Work out the finished part from the listing and answer in its coordinate system (mm). A direction names the side the tool comes from. Coordinates: 2 decimals unless noted, no trailing zeros. Loops run counter-clockwise (first coordinate to the right, second up) from the corner with the lowest first, then second, coordinate; pieces in that order, holes last. Notation, with made-up numbers: (61, 50) - (94, 50) arc R11 cw to (94, 70) - close; hole circle Ø8 at (88, -35.5). An arc over 180 degrees is marked (long way). Write each question's results on one line, items separated by ' | '. Start each with the question number.
Item 1: Section D-D, the plane y = 33.5 is taken. Write down the section's boundary in (x, z), plus the area to 3 significant figures.
Item 2: Section C-C, the plane x = -9 is taken. Write down the section's boundary in (y, z).
Item 3: Each of these flat-tipped pins is pushed along its axis until it touches: pin 1 Ø1.5 at (x, y) = (-3.5, -5.5) entering from -Z; pin 2 Ø4 at (x, y) = (0, 0) entering from +Z; pin 3 Ø1 at (x, z) = (-14.5, 3) entering from +Y; pin 4 Ø1.5 at (y, z) = (21.5, 3) entering from -X. Where does it stop, or does it pass through?
Item 4: For a pull along Y with two mould halves and no side action, classify faces 1 (the face through (0, 50, 0)), 2 (the face through (-14, -28.12, 3)), 3 (the face through (-2.476, -18.539, 1.894)) as +Y half, -Y half, draft (parallel to the pull), parting line (faces both ways), or undercut.
Item 5: Consider probe 1 along Y at (x, z) = (0, 3.2); probe 2 along Z at (x, y) = (-3, 1); probe 3 along Y at (x, z) = (-18.5, 2.05). Determine where each line is inside the solid, lowest interval first. Write a range as [from, to].
Item 6: Section A-A, the plane y = 0 is taken. Write down the section's boundary in (x, z), plus the area to 3 significant figures.
Item 7: Section B-B, the plane z = 3.4 is taken. Write down the section's boundary in (x, y).
Item 8: A tool of negligible diameter and unlimited length cuts with its end or side. For faces 4 (the face through (4, -17, 2.3)), 5 (the face through (-0.1, 9.1, 1.2)), 6 (the face through (-6.5, 31, 2)), from which of +Z, -Z, +X, -X, +Y, -Y can it reach the whole face along a straight path? Write none if from no direction.
from build123d import *

# Parameters (mm, degrees)
SKETCH1_W           = 27
SKETCH1_H           = 4
SKETCH1_W_2         = 13
SKETCH1_R           = 6.5
SKETCH1_R_2         = 2.5
BOSS_EXTRUDE1_DEPTH = 5
SKETCH2_R           = 2.5
CUT_EXTRUDE1_DEPTH  = 1.5
CUT_EXTRUDE2_DEPTH  = 0.8
FILLET1_R           = 1


with BuildPart() as part:
    # Sketch1 → Boss-Extrude1 (new body)
    # profile 1 of 6: a face of its own
    with BuildSketch(Plane.XY):
        with Locations((-20, -26.12)):
            Rectangle(SKETCH1_W, SKETCH1_H)
    # profile 2 of 6: a face of its own
    with BuildSketch(Plane.XY):
        with Locations((0, -26.12)):
            Rectangle(SKETCH1_W_2, SKETCH1_H)
    # profile 3 of 6: a face of its own
    with BuildSketch(Plane.XY):
        with BuildLine():
            Line((-6.5, -24.12), (6.5, -24.12))
            Line((6.5, -24.12), (6.5, 0))
            ThreePointArc((6.5, 0), (0, -6.5), (-6.5, 0))
            Line((-6.5, 0), (-6.5, -24.12))
        make_face()
    # profile 4 of 6: a face of its own
    with BuildSketch(Plane.XY):
        Circle(SKETCH1_R)
        Circle(SKETCH1_R_2, mode=Mode.SUBTRACT)
    # profile 5 of 6: a face of its own
    with BuildSketch(Plane.XY):
        with BuildLine():
            ThreePointArc((-6.5, 0), (0, 6.5), (6.5, 0))
            Line((6.5, 0), (6.5, 84.43))
            ThreePointArc((6.5, 84.43), (0, 77.93), (-6.5, 84.43))
            Line((-6.5, 84.43), (-6.5, 0))
        make_face()
    # profile 6 of 6: a face of its own
    with BuildSketch(Plane.XY):
        with Locations((0, 84.43)):
            Circle(SKETCH1_R)
        with Locations((0, 84.43)):
            Circle(SKETCH1_R_2, mode=Mode.SUBTRACT)
    extrude(amount=BOSS_EXTRUDE1_DEPTH)

    # Sketch2 → Cut-Extrude1 (cut)
    with BuildSketch(Plane(origin=(0, 0, 0), x_dir=(-1, 0, 0), z_dir=(0, 0, -1))):
        with BuildLine():
            Line((33.5, -28.12), (33.5, -24.12))
            Line((33.5, -24.12), (6.5, -24.12))
            Line((6.5, -24.12), (6.5, 6.368673331))
            ThreePointArc((6.5, 6.368673331), (0, 9.1), (-6.5, 6.368673331))
            Line((-6.5, 6.368673331), (-6.5, -28.12))
            Line((-6.5, -28.12), (33.5, -28.12))
        make_face()
        Circle(SKETCH2_R, mode=Mode.SUBTRACT)
    extrude(amount=-CUT_EXTRUDE1_DEPTH, mode=Mode.SUBTRACT)

    # Sketch3 → Cut-Extrude2 (cut)
    with BuildSketch(Plane(origin=(0, 0, 1.5), x_dir=(-1, 0, 0), z_dir=(0, 0, -1))):
        with BuildLine():
            ThreePointArc((-0.425, -16.56), (-1.318324317, -14.403324317), (-3.475, -13.51))
            ThreePointArc((-3.475, -13.51), (-5.489184715, -14.269681259), (-6.5, -16.170288568))
            Line((-6.5, -16.170288568), (-6.5, -16.949711432))
            ThreePointArc((-6.5, -16.949711432), (-5.489184715, -18.850318741), (-3.475, -19.61))
            ThreePointArc((-3.475, -19.61), (-1.318324317, -18.716675683), (-0.425, -16.56))
        make_face()
        with BuildLine():
            Line((-6.5, -16.949711432), (-6.5, -16.170288568))
            ThreePointArc((-6.5, -16.170288568), (-6.525, -16.56), (-6.5, -16.949711432))
        make_face()
        with BuildLine():
            Line((-6.5, -19.61), (-3.475, -19.61))
            ThreePointArc((-3.475, -19.61), (-5.489184715, -18.850318741), (-6.5, -16.949711432))
            Line((-6.5, -16.949711432), (-6.5, -19.61))
        make_face()
        with BuildLine():
            ThreePointArc((-6.5, -16.170288568), (-5.489184715, -14.269681259), (-3.475, -13.51))
            Line((-3.475, -13.51), (-6.5, -13.51))
            Line((-6.5, -13.51), (-6.5, -16.170288568))
        make_face()
        with BuildLine():
            ThreePointArc((6.5, -21.509961072), (8.002523966, -20.398869023), (8.575, -18.62))
            ThreePointArc((8.575, -18.62), (8.002523966, -16.841130977), (6.5, -15.730038928))
            Line((6.5, -15.730038928), (6.5, -21.509961072))
        make_face()
        with BuildLine():
            Line((6.5, -21.509961072), (6.5, -15.730038928))
            ThreePointArc((6.5, -15.730038928), (2.475, -18.62), (6.5, -21.509961072))
        make_face()
    extrude(amount=-CUT_EXTRUDE2_DEPTH, mode=Mode.SUBTRACT)

    # Fillet1
    fillet1_edges = [part.edges().sort_by_distance(p)[0] for p in [
        (0, 9.1, 0),
    ]]
    fillet(fillet1_edges, radius=FILLET1_R)


solid = part.part
Answer key:
1) outline: (-6.5, 0) - (6.5, 0) - (6.5, 5) - (-6.5, 5) - close | area: 65.0 mm^2
2) outline: (-28.12, 1.5) - (-24.12, 1.5) - (-24.12, 5) - (-28.12, 5) - close
3) pin 1: stops at z = 1.5 | pin 2: passes through | pin 3: stops at y = -24.12 | pin 4: stops at x = -6.5
4) face 1: draft | face 2: -Y half | face 3: undercut
5) probe 1: y = [-28.12, -2.5], [2.5, 81.93], [86.93, 90.93] | probe 2: z = [1.5, 5] | probe 3: y = [-28.12, -24.12]
6) outline: (-6.5, 1.5) - (-2.5, 1.5) - (-2.5, 5) - (-6.5, 5) - close; (2.5, 1.5) - (6.5, 1.5) - (6.5, 5) - (2.5, 5) - close | area: 28.0 mm^2
7) outline: (-33.5, -28.12) - (6.5, -28.12) - (6.5, 84.43) arc R6.5 ccw to (-6.5, 84.43) - (-6.5, -24.12) - (-33.5, -24.12) - close; hole circle Ø5 at (0, 0); hole circle Ø5 at (0, 84.43)
8) face 4: -Z, +X | face 5: -Z, -Y | face 6: +Z, -Z, -X, +Y
